Autodesk Inventor part; units mm, degrees
ref_plane "YZ Plane" through (0, 0, 0) normal (1, 0, 0) x (0, 1, 0)
ref_plane "XZ Plane" through (0, 0, 0) normal (0, 1, 0) x (-1, 0, 0)
ref_plane "XY Plane" through (0, 0, 0) normal (0, 0, 1) x (1, 0, 0)
sketch "Sketch1" plane through (0, 0, 0) normal (0, 0, 1) x (1, 0, 0)
  arc A0 (-10.36, -6.4282) -> (-8.6498, -7.1366) centre (-9.3582, -6.4282) ccw
  line L0 (-10.36, 6.4282) -> (-10.36, -6.4282)
  arc A1 (-8.6498, 7.1366) -> (-10.36, 6.4282) centre (-9.3582, 6.4282) ccw
  line L1 (-5.1567, 3.6435) -> (-8.6498, 7.1366)
  arc A2 (-4.38, 1.7684) -> (-5.1567, 3.6435) centre (-7.0317, 1.7684) ccw
  line L2 (-4.38, -1.7684) -> (-4.38, 1.7684)
  arc A3 (-5.1567, -3.6435) -> (-4.38, -1.7684) centre (-7.0317, -1.7684) ccw
  line L3 (-8.6498, -7.1366) -> (-5.1567, -3.6435)
  circle A4 centre (0, 0) radius 2.5
  line L4 (-10.5183, -12.5) -> (-4.32, -12.5)
  arc A5 (-4.32, -12.5) -> (-4.32, -10.36) centre (-4.32, -11.43) ccw
  line L5 (-4.32, -10.36) -> (-6.4282, -10.36)
  arc A6 (-7.1366, -8.6498) -> (-6.4282, -10.36) centre (-6.4282, -9.3582) ccw
  line L6 (-7.1366, -8.6498) -> (-3.6435, -5.1567)
  arc A7 (-1.7684, -4.38) -> (-3.6435, -5.1567) centre (-1.7684, -7.0317) ccw
  line L7 (-1.7684, -4.38) -> (1.7684, -4.38)
  arc A8 (3.6435, -5.1567) -> (1.7684, -4.38) centre (1.7684, -7.0317) ccw
  line L8 (3.6435, -5.1567) -> (7.1366, -8.6498)
  arc A9 (6.4282, -10.36) -> (7.1366, -8.6498) centre (6.4282, -9.3582) ccw
  line L9 (6.4282, -10.36) -> (4.32, -10.36)
  arc A10 (4.32, -10.36) -> (4.32, -12.5) centre (4.32, -11.43) ccw
  line L10 (4.32, -12.5) -> (10.5183, -12.5)
  arc A11 (10.5183, -12.5) -> (12.5, -10.5183) centre (10.5183, -10.5183) ccw
  line L11 (12.5, -10.5183) -> (12.5, -4.32)
  arc A12 (12.5, -4.32) -> (10.36, -4.32) centre (11.43, -4.32) ccw
  line L12 (10.36, -4.32) -> (10.36, -6.4282)
  arc A13 (8.6498, -7.1366) -> (10.36, -6.4282) centre (9.3582, -6.4282) ccw
  line L13 (8.6498, -7.1366) -> (5.1567, -3.6435)
  arc A14 (4.38, -1.7684) -> (5.1567, -3.6435) centre (7.0317, -1.7684) ccw
  line L14 (4.38, -1.7684) -> (4.38, 1.7684)
  arc A15 (5.1567, 3.6435) -> (4.38, 1.7684) centre (7.0317, 1.7684) ccw
  line L15 (5.1567, 3.6435) -> (8.6498, 7.1366)
  arc A16 (10.36, 6.4282) -> (8.6498, 7.1366) centre (9.3582, 6.4282) ccw
  line L16 (10.36, 6.4282) -> (10.36, 4.32)
  arc A17 (10.36, 4.32) -> (12.5, 4.32) centre (11.43, 4.32) ccw
  line L17 (12.5, 4.32) -> (12.5, 10.5183)
  arc A18 (12.5, 10.5183) -> (10.5183, 12.5) centre (10.5183, 10.5183) ccw
  line L18 (10.5183, 12.5) -> (4.32, 12.5)
  arc A19 (4.32, 12.5) -> (4.32, 10.36) centre (4.32, 11.43) ccw
  line L19 (4.32, 10.36) -> (6.4282, 10.36)
  arc A20 (7.1366, 8.6498) -> (6.4282, 10.36) centre (6.4282, 9.3582) ccw
  line L20 (7.1366, 8.6498) -> (3.6435, 5.1567)
  arc A21 (1.7684, 4.38) -> (3.6435, 5.1567) centre (1.7684, 7.0317) ccw
  line L21 (1.7684, 4.38) -> (-1.7684, 4.38)
  arc A22 (-3.6435, 5.1567) -> (-1.7684, 4.38) centre (-1.7684, 7.0317) ccw
  line L22 (-3.6435, 5.1567) -> (-7.1366, 8.6498)
  arc A23 (-6.4282, 10.36) -> (-7.1366, 8.6498) centre (-6.4282, 9.3582) ccw
  line L23 (-6.4282, 10.36) -> (-4.32, 10.36)
  arc A24 (-4.32, 10.36) -> (-4.32, 12.5) centre (-4.32, 11.43) ccw
  line L24 (-4.32, 12.5) -> (-10.5183, 12.5)
  arc A25 (-10.5183, 12.5) -> (-12.5, 10.5183) centre (-10.5183, 10.5183) ccw
  line L25 (-12.5, 10.5183) -> (-12.5, -10.5183)
  arc A26 (-12.5, -10.5183) -> (-10.5183, -12.5) centre (-10.5183, -10.5183) ccw
extrude "Extrusion1" add sketch "Sketch1" against normal blind 100
properties part number "25-2503"
Can you work these out from the model? Positions are in its coordinate system, mm. A direction names the side the tool comes from. Coordinates: 2 decimals unless noted, no trailing zeros. Order: outer loops, then holes, each group sorted by start corner. A loop starts at its lowest first (then second) coordinate and runs counter-clockwise, first axis right, second up.
1. If we section it at C-C (z = -23.5): Give the number of separate pieces and of enclosed holes in the cut face, then the cut area to 3 significant figures.
2. For faces 1 (the face through (-4.59, -2.8, -49.3)), 2 (the face through (-11.935, -11.904, -49.3)), which set-ups out of +Z, -Z, +X, -X, +Y, -Y let a thin tool reach every point of the face, with its end or its side?
3. If we section it at A-A (y = 0): Please give me the cut outline in (x, z), then the cut area to 3 significant figures.
4. If we section it at B-B (x = 0): Please give me the cut outline in (y, z).
5. Thinking about a two-plate mould opening in Y: for faces 3 (the face through (12.5, -7, -49)), 4 (the face through (-7, 12.5, -49)), 5 (the face through (3.25, 11.45, -49.3)), which applies, +Y half, -Y half, draft (parallel to the pull), parting line (faces both ways), or undercut?
6. If we section it at D-D (x = 11.43): Please give me the cut outline in (y, z), then the cut area to 3 significant figures.
7. I'm going to push flat-ended pins straight in: pin 1 (4.5 mm diameter, centred on x = 0, y = 0, fed in from -Z); pin 2 (4 mm diameter, centred on y = 0.5, z = -72.5, fed in from +X); pin 3 (4 mm diameter, centred on x = -0.5, z = -41, fed in from -Y); pin 4 (4 mm diameter, centred on x = -1.5, z = -89, fed in from -Y). Where does each tip first touch, or does it pass through?
8. I need wall thicknesses on line 1 (Y direction, x = -1.75, z = -74.5); line 2 (Y direction, x = -0.25, z = -6); line 3 (Y direction, x = 7, z = -74). Which ranges of each line are inside material? Lowest first, please.
Entries:
1. separate pieces: 1
1. enclosed holes: 2
1. area: 288 mm2
2. face 1: +Z, -Z
2. face 2: +Z, -Z, -X, -Y
3. outline: (-12.5, -100) - (-10.36, -100) - (-10.36, 0) - (-12.5, 0) - close; (-4.38, -100) - (-2.5, -100) - (-2.5, 0) - (-4.38, 0) - close; (2.5, -100) - (4.38, -100) - (4.38, 0) - (2.5, 0) - close
3. area: 590 mm2
4. outline: (-4.38, -100) - (-2.5, -100) - (-2.5, 0) - (-4.38, 0) - close; (2.5, -100) - (4.38, -100) - (4.38, 0) - (2.5, 0) - close
5. face 3: draft
5. face 4: +Y half
5. face 5: undercut
6. outline: (-12.28, -100) - (-3.25, -100) - (-3.25, 0) - (-12.28, 0) - close; (3.25, -100) - (12.28, -100) - (12.28, 0) - (3.25, 0) - close
6. area: 1,810 mm2
7. pin 1: passes through
7. pin 2: stops at x = 4.48
7. pin 3: stops at y = -4.48
7. pin 4: stops at y = -12.12
8. line 1: y = -4.38 to -1.79, 1.79 to 4.38
8. line 2: y = -4.38 to -2.49, 2.49 to 4.38
8. line 3: y = -12.5 to -10.18, -8.51 to -5.49, 5.49 to 8.51, 10.18 to 12.5
